Drawing for the job (mm, zero at the part's lowest x, y, z). A direction names the side the tool comes from. Coordinates: 2 decimals unless noted, no trailing zeros. Write each loop counter-clockwise with the first axis right and the second up, starting at its lowest first coordinate (ties: lowest second). Pieces come first, ordered by that corner, then holes. Notation, with made-up numbers: M 68,33 L 127,33 A14 cw 127,44 Z; hole C 58,41.5 d3. An arc over 180 degrees is marked long. Use CSV: the item, a comma, the result in double quotes. Start each with the question number.
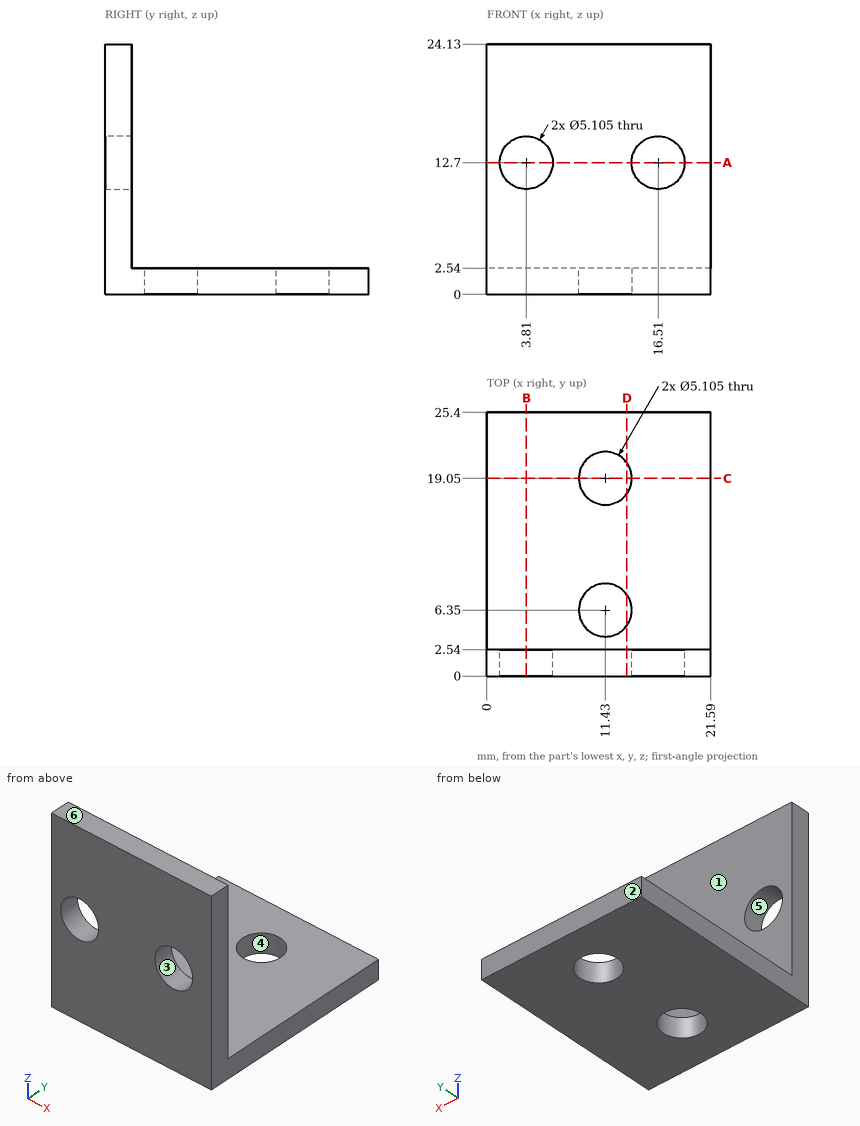
1) Wall check: L1, parallel to X at y = 1.8, z = 12.7; L2, parallel to Y at x = 11.43, z = 1.45; L3, parallel to Y at x = 6.5, z = 10. Give the ranges that are in metal, low to high. Write a range as [from, to].
2) Tool access for the marked faces 1 and 2: list every direction of +Z, -Z, +X, -X, +Y, -Y with a clear straight run to the whole face (end or side of a thin tool).
3) Band-saw the part on D-D on x = 13.5. List the corners of the cut face in (y, z), then the cut area to 3 significant figures.
4) Band-saw the part on A-A on z = 12.7. List the corners of the cut face in (x, y).
5) Two-plate mould, pull along Z, no slides. Class the marked faces 3, 4, 5 and 6: pulls with the +Z half, pulls with the -Z half, needs draft (parallel to the pull), parting line crosses it, or undercut.
6) Drop flat-ended pins along their axis: P1, Ø3, axis at x = 16.51, z = 12.7, coming from the +Y side; P2, Ø1, axis at x = 11, y = 13, coming from the -Z side; P3, Ø6.5, axis at x = 11.43, y = 6.35, coming from the +Z side; P4, Ø6, axis at x = 17, z = 10.5, coming from the +Y side. Give the stop position or say it passes through.
7) Band-saw the part on C-C on y = 19.05. List the corners of the cut face in (x, z).
8) Band-saw the part on B-B on x = 3.81. List the corners of the cut face in (y, z).
Findings below:
1,L1,"x = [0, 1.26], [6.36, 13.96], [19.06, 21.59]"
1,L2,"y = [0, 3.8], [8.9, 16.5], [21.6, 25.4]"
1,L3,"y = [0, 2.54]"
2,face 1,"+Z, +X, -X, +Y"
2,face 2,"+Z, -Z, +X, -X, +Y"
3,outline,"M 0,0 L 4.86,0 L 4.86,2.54 L 2.54,2.54 L 2.54,24.13 L 0,24.13 Z; M 7.84,0 L 17.56,0 L 17.56,2.54 L 7.84,2.54 Z; M 20.54,0 L 25.4,0 L 25.4,2.54 L 20.54,2.54 Z"
3,area,"104 mm2"
4,outline,"M 0,0 L 1.26,0 L 1.26,2.54 L 0,2.54 Z; M 6.36,0 L 13.96,0 L 13.96,2.54 L 6.36,2.54 Z; M 19.06,0 L 21.59,0 L 21.59,2.54 L 19.06,2.54 Z"
5,face 3,"undercut"
5,face 4,"needs draft"
5,face 5,"undercut"
5,face 6,"pulls with the +Z half"
6,P1,"passes through"
6,P2,"stops at z = 0"
6,P3,"stops at z = 2.54"
6,P4,"stops at y = 2.54"
7,outline,"M 0,0 L 8.88,0 L 8.88,2.54 L 0,2.54 Z; M 13.98,0 L 21.59,0 L 21.59,2.54 L 13.98,2.54 Z"
8,outline,"M 0,0 L 25.4,0 L 25.4,2.54 L 2.54,2.54 L 2.54,10.15 L 0,10.15 Z; M 0,15.25 L 2.54,15.25 L 2.54,24.13 L 0,24.13 Z"
